```python
from build123d import *

# Parameters (mm, degrees)
FILETE4_R             = 5
FILETE5_R             = 2
FILETE6_R             = 2
ESBO_O2_R             = 3
CORTE_EXTRUS_O1_DEPTH = 6
PADR_OCIRCULAR1_COUNT = 8
CHANFRO3_SIZE         = 3
CHANFRO3_SIZE2        = 1.391688553


with BuildPart() as part:
    # Esboço1 → Revolução1 (revolve)
    with BuildSketch(Plane.XY, mode=Mode.PRIVATE) as revolu_o1_sk:
        Polygon((-13.688060187, 0), (-16.688060187, 0), (-16.688060187, -6), (-13.888060187, -6), (-13.888060187, -9.5), (-16.688060187, -9.5), (-16.688060187, -30), (6.757041151, -56.954385068), (-3.162394771, -132.299981266), (-0.188060187, -132.691559843), (9.811939813, -56.734018716), align=None)
    revolve(revolu_o1_sk.sketch.rotate(Axis((17.811939813, -4.773902368, 0), (0, 1, 0)), 270), axis=Axis((17.811939813, -4.773902368, 0), (0, 1, 0)))

    # Filete4
    filete4_edges = [part.edges().sort_by_distance(p)[0] for p in [
        (17.811939813, -56.954385068, 11.054898662),
    ]]
    fillet(filete4_edges, radius=FILETE4_R)

    # Filete5
    filete5_edges = [part.edges().sort_by_distance(p)[0] for p in [
        (17.811939813, -132.299981266, 20.974334584),
    ]]
    fillet(filete5_edges, radius=FILETE5_R)

    # Filete6
    filete6_edges = [part.edges().sort_by_distance(p)[0] for p in [
        (17.811939813, -56.734018716, 8),
    ]]
    fillet(filete6_edges, radius=FILETE6_R)

    # Esboço2 → Corte-extrusão1 (cut)
    with BuildSketch(Plane.XY.offset(-34.5)):
        with Locations(Location((17.811939813, -20, 0), (0, 0, 270))):
            Circle(ESBO_O2_R)
    corte_extrus_o1 = extrude(amount=CORTE_EXTRUS_O1_DEPTH, mode=Mode.SUBTRACT)

    # PadrãoCircular1: Corte-extrusão1 ×8 about axis
    padr_ocircular1_axis = Axis((17.811939813, 0, 0), (0, 1, 0))
    for i in range(1, PADR_OCIRCULAR1_COUNT):
        add(corte_extrus_o1.rotate(padr_ocircular1_axis, i * 360 / PADR_OCIRCULAR1_COUNT), mode=Mode.SUBTRACT)

    # Chanfro3
    chanfro3_edges = [part.edges().sort_by_distance(p)[0] for p in [
        (17.811939813, 0, 31.5),
    ]]
    chanfro3_side = [part.faces().sort_by_distance(p)[0] for p in [
        (17.811939813, -28.119456583, 19.852539717),
    ]]
    chamfer(chanfro3_edges, length=CHANFRO3_SIZE, length2=CHANFRO3_SIZE2, reference=chanfro3_side[0])


solid = part.part
```
Input: part model. Units: mm. Frame: model coordinates. A direction names the side the tool comes from. Give positions to 0.01 mm unless a question says otherwise; leave off trailing zeros. Loops run counter-clockwise (first coordinate to the right, second up) from the corner with the lowest first, then second, coordinate; pieces in that order, holes last.
1) Reachability of faces 1 (the flat face through (18, -20, 28.5)), 2 (the conical face through (36.38, -2.6, 24.21)), 3 (the cylindrical face through (14.883, -19.35, -31.542)), 4 (the conical face through (26.09, -54.03, 10.79)), 5 (the flat face through (46.312, -20, 0)) from +Z, -Z, +X, -X, +Y, -Y: full face, straight path, thin tool, end or side. Return the list, or none.
A:
face 1: +Z
face 2: +Y
face 3: -Z
face 4: none
face 5: +X
2) Mould query, pull axis Z, two halves, no side actions, for faces 6 (the conical face through (22.778, -94.45, -11.977)), 7 (the cylindrical face through (37.101, -7.774, 25.156)), 8 (the cylindrical face through (-14, -17, 0)), 9 (the flat face through (30, 0, 31)). Classes: released by +Z, released by -Z, zero draft, split by the parting line, or undercut.
A:
face 6: undercut
face 7: split by the parting line
face 8: undercut
face 9: zero draft
3) Line query: L1, parallel to Z at x = -2.5, y = -20.5; L2, parallel to X at y = -17.5, z = 1.5; L3, parallel to Z at x = 18, y = -65.5. Output: solid intervals per line, ascending.
A:
L1: z = -27.89 to -24.5, -19.99 to -10.81, 10.81 to 19.99, 24.5 to 27.89
L2: x = -10.69 to -6.39, 42.02 to 46.31
L3: z = -12.18 to -9.15, 9.15 to 12.18
4) Contact query for flat-ended pins moving along their axis: pin 1 (5 mm diameter, centred on x = 17, y = -20, fed in from +Z); pin 2 (8 mm diameter, centred on x = 17.81, y = -20, fed in from +Z); pin 3 (12 mm diameter, centred on x = 17.5, y = -77.5, fed in from +Z); pin 4 (3 mm diameter, centred on y = -40.5, z = -0.5, fed in from +X). Output: stop coordinate, or through.
A:
pin 1: stops at z = 34.44
pin 2: stops at z = 34.5
pin 3: stops at z = 14.55
pin 4: stops at x = 44.48
5) Section query B-B on y = -92.5. Return the cut outline in (x, z), and give its area (3 significant figures).
A:
outline: circle Ø31.47 at (17.81, 0); hole circle Ø25.42 at (17.81, 0)
area: 270 mm2
6) Section query C-C on y = -120.5. Return the cut outline in (x, z).
A:
outline: circle Ø38.84 at (17.81, 0); hole circle Ø32.79 at (17.81, 0)
